Can you work these out from the model? Positions are in its coordinate system, mm. A direction names the side the tool comes from. Give positions to 0.01 mm unless a question says otherwise; leave off trailing zeros. Write each loop counter-clockwise with the first axis right and the second up, starting at its lowest first coordinate (ties: lowest second). Pieces come first, ordered by that corner, then holes.
from build123d import *

# Parameters (mm, degrees)
F1_DEPTH  = 25.4
F2_W      = 27.94
F2_H      = 12.446
F3_DEPTH  = 25.4
F4_R      = 5.715
F5_DEPTH  = 25.4
F6_W      = 25.4
F6_H      = 50.8
F7_DEPTH  = 25.4
F8_R      = 6.096
F10_DEPTH = 25.4


with BuildPart() as f1:
    # F0 (on Front) → F1 (new body)
    with BuildSketch(Plane.XZ):
        Polygon((-12.7, -49.002826), (0, -49.002826), (12.7, -49.002826), (12.7, 1.797174), (-12.7, 1.797174), align=None)
    extrude(amount=F1_DEPTH)

    # F2 (on face) → F3 (join)
    with BuildSketch(Plane(origin=(-12.7, 0, 0), x_dir=(0, -1, 0), z_dir=(-1, 0, 0))):
        with Locations((39.37, -4.425826)):
            Rectangle(F2_W, F2_H)
        with Locations((39.37, -42.779826)):
            Rectangle(F2_W, F2_H)
    extrude(amount=-F3_DEPTH)

    # F4 (on face) → F5 (join)
    with BuildSketch(Plane(origin=(0, 0, 0), x_dir=(-1, 0, 0), z_dir=(0, 1, 0))):
        with Locations((0, -23.602826)):
            Circle(F4_R)
    extrude(amount=F5_DEPTH)

    # F6 (on face) → F7 (join)
    with BuildSketch(Plane.XZ.offset(53.34)):
        with Locations((0, -23.602826)):
            Rectangle(F6_W, F6_H)
    extrude(amount=F7_DEPTH)

    # F8
    f8_edges = [f1.edges().sort_by_distance(p)[0] for p in [
        (-12.7, 0, -23.602826),
        (12.7, 0, -23.602826),
        (0, 0, 1.797174),
        (0, 0, -49.002826),
        (-12.7, -39.37, -36.556826),
        (-12.7, -39.37, -10.648826),
        (12.7, -39.37, -36.556826),
        (12.7, -39.37, -10.648826),
        (-12.7, -39.37, 1.797174),
        (12.7, -39.37, 1.797174),
        (12.7, -39.37, -49.002826),
        (-12.7, -39.37, -49.002826),
        (-12.7, -25.4, -23.602826),
        (12.7, -25.4, -23.602826),
        (0, -78.74, 1.797174),
        (0, -78.74, -49.002826),
        (-12.7, -78.74, -23.602826),
        (12.7, -78.74, -23.602826),
        (-12.7, -53.34, -23.602826),
        (12.7, -53.34, -23.602826),
    ]]
    fillet(f8_edges, radius=F8_R)

    # F9 (on face) → F10 (join)
    with BuildSketch(Plane.XZ.offset(78.74)):
        with BuildLine():
            ThreePointArc((5.715, -23.602826), (4.041115, -19.561711), (0, -17.887826))
            Line((0, -17.887826), (0, -23.602826))
            Line((0, -23.602826), (0, -29.317826))
            ThreePointArc((0, -29.317826), (4.041115, -27.643941), (5.715, -23.602826))
        make_face()
        with BuildLine():
            Line((0, -23.602826), (0, -17.887826))
            ThreePointArc((0, -17.887826), (-5.715, -23.602826), (0, -29.317826))
            Line((0, -29.317826), (0, -23.602826))
        make_face()
    extrude(amount=F10_DEPTH)


solid = f1.part
(1) Imagine slicing it at A-A, the plane z = -35. Write out the boundary of the cut face in (x, y), plus the area to 3 significant figures.
Returned:
outline: (-12.7, -72.64) arc R6.1 ccw to (-6.6, -78.74) - (6.6, -78.74) arc R6.1 ccw to (12.7, -72.64) - (12.7, -59.44) arc R6.1 ccw to (6.6, -53.34) - (-6.6, -53.34) arc R6.1 ccw to (-12.7, -59.44) - close; (-12.7, -19.3) arc R6.1 ccw to (-6.6, -25.4) - (6.6, -25.4) arc R6.1 ccw to (12.7, -19.3) - (12.7, -6.1) arc R6.1 ccw to (6.6, 0) - (-6.6, 0) arc R6.1 ccw to (-12.7, -6.1) - close
area: 1,230 mm2
(2) If I drill on L1, parallel to Y at x = -1.25, z = -12; L2, parallel to Y at x = 3, z = -19; L3, parallel to Y at x = 0.5, z = -41.5, over which ranges is the centre line in solid material (lowest first)?
Returned:
L1: y = -78.74 to -53.34, -25.4 to 0
L2: y = -104.14 to -53.34, -25.4 to 25.4
L3: y = -78.74 to 0
(3) Imagine slicing it at C-C, the plane x = -3.5. Write out the boundary of the cut face in (y, z), plus the area to 3 significant figures.
Returned:
outline: (-104.14, -28.12) - (-78.74, -28.12) - (-78.74, -42.91) arc R6.1 ccw to (-72.64, -49) - (-6.1, -49) arc R6.1 ccw to (0, -42.91) - (0, -28.12) - (25.4, -28.12) - (25.4, -19.08) - (0, -19.08) - (0, -4.3) arc R6.1 ccw to (-6.1, 1.8) - (-72.64, 1.8) arc R6.1 ccw to (-78.74, -4.3) - (-78.74, -19.08) - (-104.14, -19.08) - close; hole (-53.34, -36.56) - (-25.4, -36.56) - (-25.4, -10.65) - (-53.34, -10.65) - close
area: 3,700 mm2
(4) If we mould it in two halves opening along Z, with no side actions, what happens to faces 5 (the face through (0, 25.4, -24)), 6 (the face through (0, -39, -10.649)), 7 (the face through (1.24, 12.52, -29.18))? For each: +Z half, -Z half, draft (parallel to the pull), parting line (faces both ways), or undercut.
Returned:
face 5: draft
face 6: undercut
face 7: parting line
(5) Imagine slicing it at D-D, the plane y = -16. Write out the boundary of the cut face in (x, z), plus the area to 3 significant figures.
Returned:
outline: (-12.7, -42.91) arc R6.1 ccw to (-6.6, -49) - (6.6, -49) arc R6.1 ccw to (12.7, -42.91) - (12.7, -4.3) arc R6.1 ccw to (6.6, 1.8) - (-6.6, 1.8) arc R6.1 ccw to (-12.7, -4.3) - close
area: 1,260 mm2
(6) Will these pins go through, and if not, where does the flat tip stop? P1, Ø4, axis at y = -90.5, z = -28, coming from the +X side; P2, Ø3, axis at x = -5, z = -9.5, coming from the -Y side; P3, Ø1, axis at y = -5, z = -34, coming from the +X side.
Returned:
P1: stops at x = 5.19
P2: stops at y = -78.74
P3: stops at x = 12.67
(7) For faces 1 (the face through (0.09, -76.91, -47.26)), 2 (the face through (10.96, -23.57, -23.34)), 3 (the face through (-10.96, -39.65, -38.39)), 4 (the face through (0, -53.34, -23)), which set-ups out of +Z, -Z, +X, -X, +Y, -Y let a thin tool reach every point of the face, with its end or its side?
Returned:
face 1: -Z, +X, -X, -Y
face 2: +X
face 3: -X
face 4: +X, -X
(8) Imagine slicing it at B-B, the plane y = -41.5. Write out the boundary of the cut face in (x, z).
Returned:
outline: (-12.7, -42.91) arc R6.1 ccw to (-6.6, -49) - (6.6, -49) arc R6.1 ccw to (12.7, -42.91) - (12.7, -42.65) arc R6.1 ccw to (6.6, -36.56) - (-6.6, -36.56) arc R6.1 ccw to (-12.7, -42.65) - close; (-12.7, -4.55) arc R6.1 ccw to (-6.6, -10.65) - (6.6, -10.65) arc R6.1 ccw to (12.7, -4.55) - (12.7, -4.3) arc R6.1 ccw to (6.6, 1.8) - (-6.6, 1.8) arc R6.1 ccw to (-12.7, -4.3) - close
